Could you check a few things on this drawing? It's one solid part, dimensions in mm from its lowest x, y, z. Coordinates: 2 decimals unless noted, no trailing zeros. Order: outer loops, then holes, each group sorted by start corner. A loop starts at its lowest first (then second) coordinate and runs counter-clockwise, first axis right, second up.
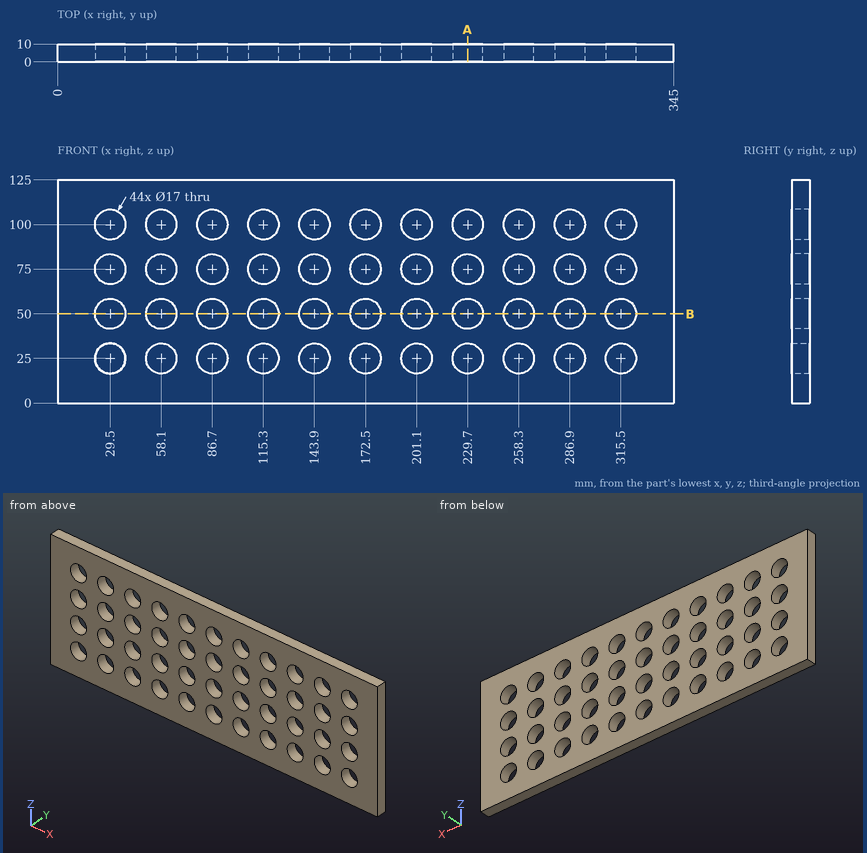
Item 1: I need wall thicknesses on line 1 (Z direction, x = 172.5, y = 4.5); line 2 (Z direction, x = 206.5, y = 5). Which ranges of each line are inside material? Lowest first, please.
Item 2: Suppose I cut it at A-A (x = 229.7). List the corners of the cut face in (y, z) for me, and give its area (3 significant figures).
Item 3: For pin 1 Ø13.5 at (x, z) = (172.5, 25) entering from -Y, with a flat end and sliding along its axis, tell me the tip position at first contact or that it passes through.
Item 4: Suppose I cut it at B-B (z = 50). Count the separate pieces of the cut face and the enclosed holes in it, and give its area (3 significant figures).
Geometry results:
1. line 1: z = 0 to 16.5, 33.5 to 41.5, 58.5 to 66.5, 83.5 to 91.5, 108.5 to 125
1. line 2: z = 0 to 18.44, 31.56 to 43.44, 56.56 to 68.44, 81.56 to 93.44, 106.56 to 125
2. outline: (0, 0) - (10, 0) - (10, 16.5) - (0, 16.5) - close; (0, 33.5) - (10, 33.5) - (10, 41.5) - (0, 41.5) - close; (0, 58.5) - (10, 58.5) - (10, 66.5) - (0, 66.5) - close; (0, 83.5) - (10, 83.5) - (10, 91.5) - (0, 91.5) - close; (0, 108.5) - (10, 108.5) - (10, 125) - (0, 125) - close
2. area: 570 mm2
3. pin 1: passes through
4. separate pieces: 12
4. enclosed holes: 0
4. area: 1,580 mm2
